Input: part model. Units: mm. Frame: model coordinates. A direction names the side the tool comes from. Give positions to 0.01 mm unless a question says otherwise; leave off trailing zeros. Write each loop counter-clockwise with the first axis right and the second up, starting at its lowest first coordinate (ties: lowest second). Pieces come first, ordered by that corner, then holes. Notation, with made-up numbers: (72, 66) - (81, 66) arc R23 ccw to (81, 100) - close; hole circle Ø6 at (71, -15.75). An arc over 180 degrees is marked (long way). Answer as a JSON object with one key per item and string values. Group by question number.
from build123d import *

# Parameters (mm, degrees)
CYLINDER005_R     = 1.95
CYLINDER005_DEPTH = 4.3
CYLINDER006_R     = 3.5
CYLINDER006_DEPTH = 2.8


with BuildPart() as cylinder005:
    # Cylinder005 → Cylinder005 (new body)
    with BuildSketch(Plane.XY):
        Circle(CYLINDER005_R)
    extrude(amount=CYLINDER005_DEPTH)


with BuildPart() as obj1:
    # Cylinder006 → Cylinder006 (new body)
    with BuildSketch(Plane.XY):
        Circle(CYLINDER006_R)
    extrude(amount=CYLINDER006_DEPTH)

    # Fusion002: union Cylinder005
    add(cylinder005.part)


with BuildPart() as obj1_1:
    # Fusion002 placement: moved
    add(obj1.part.moved(Location((-41, 0, 0))))


solid = obj1_1.part
1) Cut plane A-A on y = 0. Return the cut outline in (x, z), and give its area (4 significant figures).
2) Pin query (flat end, axial travel): P1, Ø1, axis at y = 2, z = 3, coming from the -X side; P2, Ø1, axis at y = -1.5, z = 2, coming from the -X side. Return the tip coordinate at first contact, or that it passes through.
3) Cut plane C-C on z = 3.5. Return the cut outline in (x, y), and give its area (3 significant figures).
4) Line query: line 1 along Z through (x, y) = (-38.5, 1); line 2 along Y through (x, z) = (-44, 0.55); line 3 along X through (y, z) = (0.5, 1.1). Output: solid intervals per line, ascending. Write a range as from..to.
5) Cut plane D-D on z = 1.05. Return the cut outline in (x, y).
6) Reachability of faces 1 (the face through (-44.497, 0.154, 1.38)), 2 (the face through (-39, -2, 2.8)) from +Z, -Z, +X, -X, +Y, -Y: full face, straight path, thin tool, end or side. Return the list, or none.
7) Cut plane B-B on x = -41. Return the cut outline in (y, z), and give its area (4 significant figures).
Filled in:
{
 "1": {"outline": "(-44.5, 0) - (-37.5, 0) - (-37.5, 2.8) - (-39.05, 2.8) - (-39.05, 4.3) - (-42.95, 4.3) - (-42.95, 2.8) - (-44.5, 2.8) - close", "area": "25.45 mm²"},
 "2": {"P1": "stops at x = -44.14", "P2": "stops at x = -44.35"},
 "3": {"outline": "circle Ø3.9 at (-41, 0)", "area": "11.9 mm²"},
 "4": {"line 1": "z = 0..2.8", "line 2": "y = -1.8..1.8", "line 3": "x = -44.46..-37.54"},
 "5": {"outline": "circle Ø7 at (-41, 0)"},
 "6": {"face 1": "+Z, -Z", "face 2": "+Z"},
 "7": {"outline": "(-3.5, 0) - (3.5, 0) - (3.5, 2.8) - (1.95, 2.8) - (1.95, 4.3) - (-1.95, 4.3) - (-1.95, 2.8) - (-3.5, 2.8) - close", "area": "25.45 mm²"}
}
